Answer from the drawing. Dimensions are ordinates in mm from the lowest x, y and z of the part. A direction names the side the tool comes from. Round coordinates to 2 decimals unless told otherwise and drop trailing zeros. Write each loop counter-clockwise with the first axis right and the second up, starting at its lowest first coordinate (ties: lowest second). Pieces come first, ordered by that corner, then holes. Notation, with made-up numbers: (-11.5, 6) - (-3.5, 6) arc R22 ccw to (-3.5, 21) - close; hole circle Ø2 at (46.25, 12). An arc over 180 degrees is marked (long way). Answer as CSV lines item,"result". Start each with the question number.
1) Which of the six approach directions +Z, -Z, +X, -X, +Y, -Y give full straight-line access (tool end or side, diameter ignored) to the marked faces 5 and 6?
2) Each of these flat-tipped pins is pushed along its axis until it touches: pin 1 (2 mm diameter, centred on x = 24, y = 80.5, fed in from +Z); pin 2 (3 mm diameter, centred on x = 32, y = 114, fed in from -Z) (1 decimal); pin 3 (2 mm diameter, centred on x = 42, z = 11, fed in from -Y); pin 4 (8 mm diameter, centred on x = 19.5, y = 83, fed in from +Z). Where does it stop, or does it pass through?
3) Find section C-C on y = 42.5. Determine the outline of the cut face in (x, z) (1 decimal), then the cut area to 3 significant figures.
4) Consider line 1 along X through (y, z) = (49.5, 31.5); line 2 along Z through (x, y) = (20, 77) (1 decimal); line 3 along Z through (x, y) = (31.5, 49) (1 decimal). Determine where each line is inside the solid, lowest interval first.
5) Find section B-B on y = 87. Determine the outline of the cut face in (x, z) (1 decimal).
6) For a pull along X with two mould halves and no side action, classify the marked faces 1, 2, 3 and 4 as +X half, -X half, draft (parallel to the pull), parting line (faces both ways), or undercut.
7) Find section A-A on x = 25.4. Determine the outline of the cut face in (y, z) (1 decimal), then the cut area to 3 significant figures.
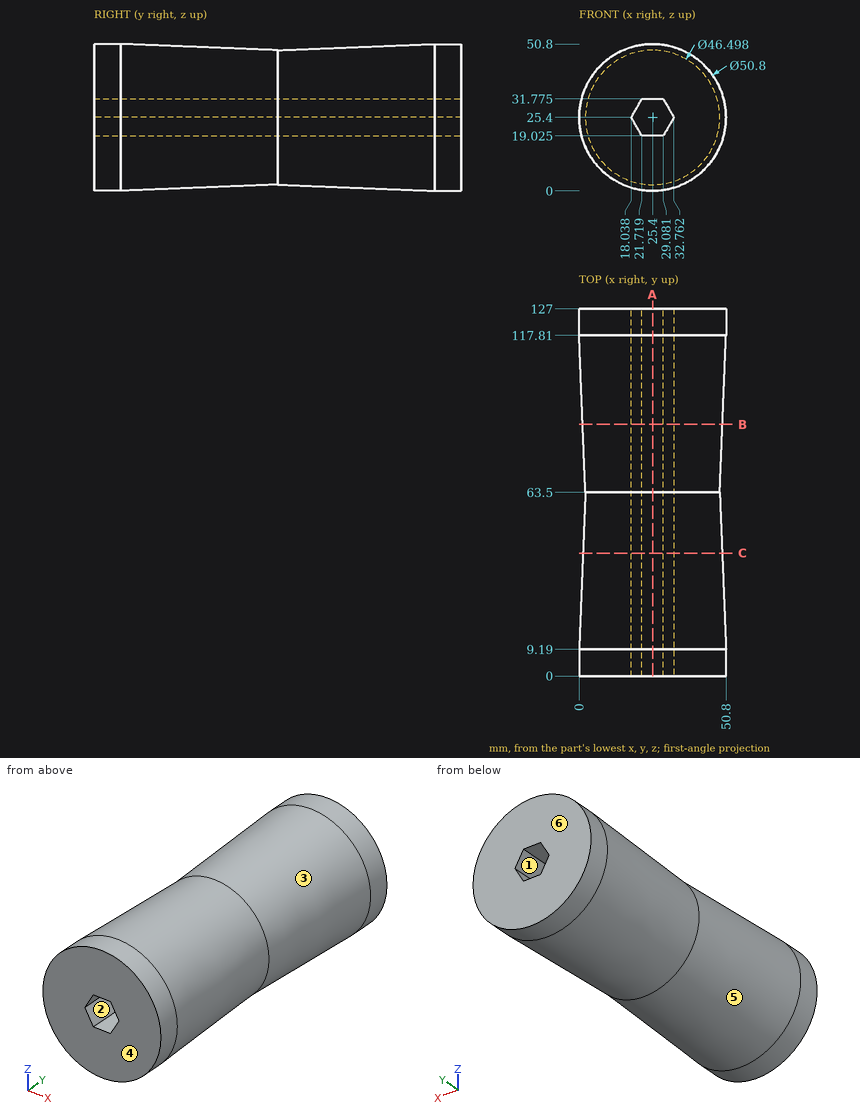
Check values:
1,face 5,"none"
1,face 6,"+Z, -Z, +X, -X, +Y"
2,pin 1,"stops at z = 49.34"
2,pin 2,"stops at z = 0.7"
2,pin 3,"stops at y = 0"
2,pin 4,"stops at z = 49.38"
3,outline,"circle Ø48.2 at (25.4, 25.4); hole (18, 25.4) - (21.7, 19) - (29.1, 19) - (32.8, 25.4) - (29.1, 31.8) - (21.7, 31.8) - close"
3,area,"1,680 mm^2"
4,line 1,"x = 2.39 to 21.56, 29.24 to 48.41"
4,line 2,"z = 2.2 to 22, 28.8 to 48.6"
4,line 3,"z = 2.4 to 23.2, 27.6 to 48.4"
5,outline,"circle Ø48.4 at (25.4, 25.4); hole (18, 25.4) - (21.7, 19) - (29.1, 19) - (32.8, 25.4) - (29.1, 31.8) - (21.7, 31.8) - close"
6,face 1,"undercut"
6,face 2,"undercut"
6,face 3,"parting line"
6,face 4,"draft"
7,outline,"(0, 0) - (9.2, 0) - (63.5, 2.2) - (117.8, 0) - (127, 0) - (127, 19) - (0, 19) - close; (0, 31.8) - (127, 31.8) - (127, 50.8) - (117.8, 50.8) - (63.5, 48.6) - (9.2, 50.8) - (0, 50.8) - close"
7,area,"4,600 mm^2"
